from build123d import *

# Parameters (mm, degrees)
CHAMFER1_SIZE = 0.254


with BuildPart() as part:
    # Sketch1 → Revolve1 (revolve)
    with BuildSketch(Plane.XY, mode=Mode.PRIVATE) as revolve1_sk:
        Polygon((-3.9624, 0), (-3.1877, 0), (-3.1877, -25.4), (-6.096, -25.4), (-8.636, -22.86), (-8.636, -21.336), (-6.096, -18.796), (-5.207, -8.634683503), (-5.207, -1.2446), align=None)
    revolve(revolve1_sk.sketch.rotate(Axis((0, 0, 0), (0, -1, 0)), 270), axis=Axis((0, 0, 0), (0, -1, 0)))

    # Chamfer1
    chamfer1_edges = [part.edges().sort_by_distance(p)[0] for p in [
        (0, 0, -3.1877),
        (0, -25.4, -3.1877),
    ]]
    chamfer(chamfer1_edges, length=CHAMFER1_SIZE)


solid = part.part
Verification items for the finished model (mm, model axes). A direction names the side the tool comes from. Coordinates: 2 decimals unless noted, no trailing zeros. Order: outer loops, then holes, each group sorted by start corner. A loop starts at its lowest first (then second) coordinate and runs counter-clockwise, first axis right, second up.
Item 1: Section check D-D, the plane y = -16. Enter the section's corners in (x, z), then the cut area to 3 significant figures.
Filled in:
outline: circle Ø11.7 at (0, 0); hole circle Ø6.38 at (0, 0)
area: 75.6 mm2
Item 2: Material ranges on L1, parallel to X at y = -6.75, z = 0; L2, parallel to Z at x = 2, y = -21.5; L3, parallel to X at y = -16.25, z = 2.75, recorded low to high.
Filled in:
L1: x = -5.21 to -3.19, 3.19 to 5.21
L2: z = -8.4 to -2.48, 2.48 to 8.4
L3: x = -5.19 to -1.61, 1.61 to 5.19
Item 3: Access from +Z, -Z, +X, -X, +Y, -Y to the whole of each face (thin tool, end or side, straight path). Record for faces 4 (the face through (-1.564, -4.888, 4.967)), 5 (the face through (-1.9, -25.2, 6)).
Filled in:
face 4: +Y
face 5: -Y
Item 4: Section check C-C, the plane y = -7. Enter the section's corners in (x, z).
Filled in:
outline: circle Ø10.41 at (0, 0); hole circle Ø6.38 at (0, 0)
Item 5: Section check A-A, the plane x = 0. Enter the section's corners in (y, z), then the cut area to 3 significant figures.
Filled in:
outline: (-25.4, -6.1) - (-22.86, -8.64) - (-21.34, -8.64) - (-18.8, -6.1) - (-8.63, -5.21) - (-1.24, -5.21) - (0, -3.96) - (0, -3.44) - (-0.25, -3.19) - (-25.15, -3.19) - (-25.4, -3.44) - close; (-25.4, 3.44) - (-25.15, 3.19) - (-0.25, 3.19) - (0, 3.44) - (0, 3.96) - (-1.24, 5.21) - (-8.63, 5.21) - (-18.8, 6.1) - (-21.34, 8.64) - (-22.86, 8.64) - (-25.4, 6.1) - close
area: 142 mm2
Item 6: Section check B-B, the plane z = 0. Enter the section's corners in (x, y), then the cut area to 3 significant figures.
Filled in:
outline: (-8.64, -22.86) - (-6.1, -25.4) - (-3.44, -25.4) - (-3.19, -25.15) - (-3.19, -0.25) - (-3.44, 0) - (-3.96, 0) - (-5.21, -1.24) - (-5.21, -8.63) - (-6.1, -18.8) - (-8.64, -21.34) - close; (3.19, -25.15) - (3.44, -25.4) - (6.1, -25.4) - (8.64, -22.86) - (8.64, -21.34) - (6.1, -18.8) - (5.21, -8.63) - (5.21, -1.24) - (3.96, 0) - (3.44, 0) - (3.19, -0.25) - close
area: 142 mm2
Item 7: Release check for a two-part mould opening along Z. For faces 1 (the face through (3, -25.4, -3)), 2 (the face through (-8.563, -22.087, -1.124)), 3 (the face through (1.221, -12.874, 2.945)) record: +Z half, -Z half, draft (parallel to the pull), parting line (faces both ways), or undercut.
Filled in:
face 1: draft
face 2: parting line
face 3: undercut
Item 8: Depth check by flat-ended pin: pin 1 (1 mm diameter, centred on x = 6, y = -10.5, fed in from -Z); pin 2 (8 mm diameter, centred on y = -6.5, z = 0, fed in from -X); pin 3 (4 mm diameter, centred on x = 3, y = -15, fed in from -Z); pin 4 (4 mm diameter, centred on y = -19, z = -0.5, fed in from -X). Enter the tip coordinate at first touch or a pass-through.
Filled in:
pin 1: passes through
pin 2: stops at x = -5.37
pin 3: stops at z = -5.72
pin 4: stops at x = -8.29
